The figure shows three views and two pictorial views of one solid part (mm, origin at its lowest corner). Answer the questions. Give positions to 0.01 mm unless a question says otherwise; leave off trailing zeros. Order: outer loops, then holes, each group sorted by start corner. A loop starts at its lowest first (then second) coordinate and runs counter-clockwise, first axis right, second up. Notation, with made-up numbers: (22, 31.25) - (78, 31.25) arc R21 ccw to (78, 47.25) - close; hole circle Ø7 at (22, 29.5). An arc over 180 degrees is marked (long way). Use a Markdown table: item, result. Add a question column.
1. A cutting plane is placed at B-B on z = 157. Determine the outline of the cut face in (x, y).
2. A cutting plane is placed at A-A on y = 6. Determine the outline of the cut face in (x, z).
3. A cutting plane is placed at D-D on z = 226. Determine the outline of the cut face in (x, y).
4. Consider L1, parallel to Z at x = 198, y = 18; L2, parallel to Y at x = 312.5, z = 458; L3, parallel to X at y = 16, z = 158. Determine where each line is inside the solid, lowest interval first.
5. For a pull along Z with two mould halves and no side action, classify the marked faces 1 and 2 as released by +Z, released by -Z, zero draft, split by the parting line, or undercut.
6. A cutting plane is placed at C-C on x = 184.5. Determine the outline of the cut face in (y, z), and give its area (3 significant figures).
7. Flat-ended cylindrical pins translate along their axes: P1, Ø16, axis at y = 11.5, z = 60, coming from the -X side; P2, Ø4, axis at x = 296, y = 9, coming from the +Z side; P3, Ø3, axis at x = 201.5, z = 367, coming from the -Y side. Find the tip coordinate at first contact, or state that the pin passes through.
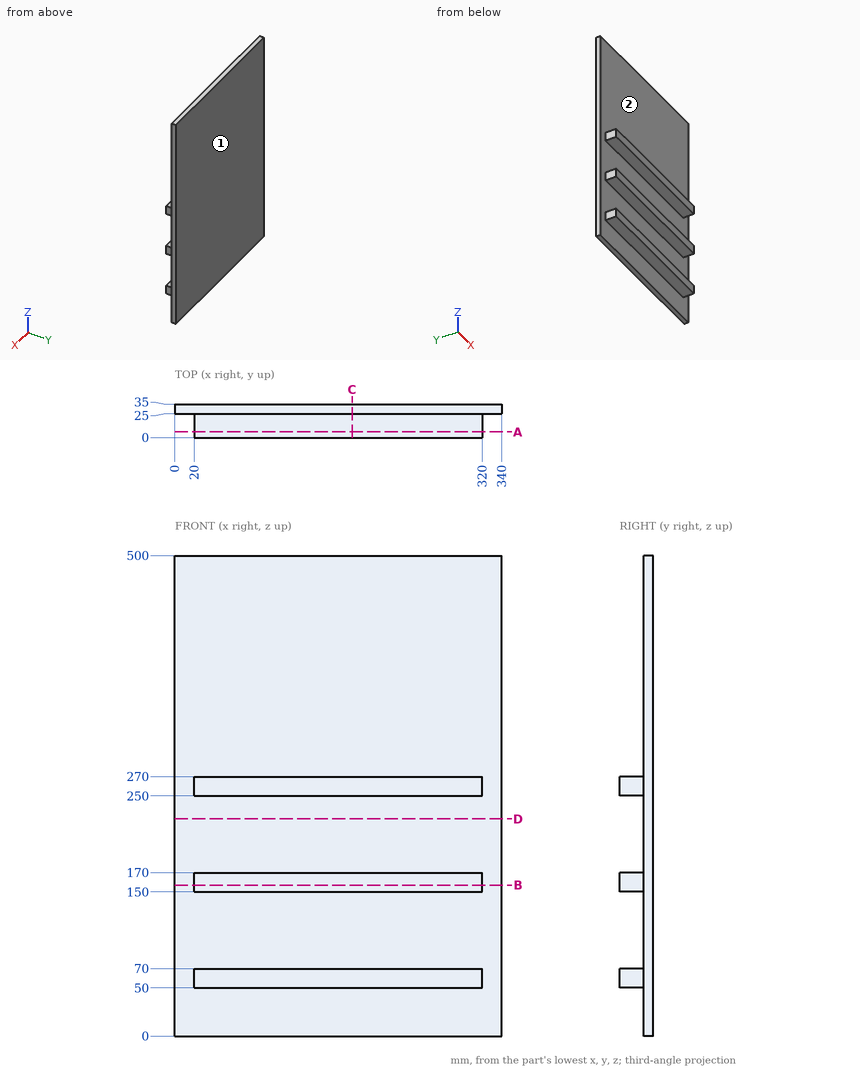
Output values:
| question | item | result |
|---|---|---|
| 1 | outline | (0, 25) - (20, 25) - (20, 0) - (320, 0) - (320, 25) - (340, 25) - (340, 35) - (0, 35) - close |
| 2 | outline | (20, 50) - (320, 50) - (320, 70) - (20, 70) - close; (20, 150) - (320, 150) - (320, 170) - (20, 170) - close; (20, 250) - (320, 250) - (320, 270) - (20, 270) - close |
| 3 | outline | (0, 25) - (340, 25) - (340, 35) - (0, 35) - close |
| 4 | L1 | 50 to 70, 150 to 170, 250 to 270 |
| 4 | L2 | 25 to 35 |
| 4 | L3 | 20 to 320 |
| 5 | face 1 | zero draft |
| 5 | face 2 | undercut |
| 6 | outline | (0, 50) - (25, 50) - (25, 0) - (35, 0) - (35, 500) - (25, 500) - (25, 270) - (0, 270) - (0, 250) - (25, 250) - (25, 170) - (0, 170) - (0, 150) - (25, 150) - (25, 70) - (0, 70) - close |
| 6 | area | 6,500 mm² |
| 7 | P1 | x = 20 |
| 7 | P2 | z = 270 |
| 7 | P3 | y = 25 |
